Build history of the part. All positions in model axes, mm. A direction names the side the tool comes from. Round coordinates to 2 decimals unless told otherwise and drop trailing zeros. Write each loop counter-clockwise with the first axis right and the second up, starting at its lowest first coordinate (ties: lowest second). Pieces come first, ordered by that corner, then holes. Notation, with made-up numbers: M -1,64 L 40,64 A23 cw 40,82 Z; hole C 15.5,-25.5 d11. An arc over 180 degrees is marked long. Write item = value, one per line. Start each with the question number.
Q1. Band-saw the part on A-A on z = 0. Write the cut outline in (x, y).
Q2. Drop flat-ended pins along their axis: P1, Ø1, axis at x = 7.5, y = -2.5, coming from the -Z side; P2, Ø1.5, axis at x = 16, z = -2, coming from the -Y side; P3, Ø4, axis at x = -12.5, y = -11, coming from the +Z side. Give the stop position or say it passes through.
Q3. Pull direction Y, two halves, no side cores. Call faces 6 (the flat face through (0, 10, 0)), 7 (the cylindrical face through (-15.5, 0.1, 0)), 8 (the cylindrical face through (10.5, 0.1, 0)), 9 (the flat face through (0, 0, -2)): released by +Y, released by -Y, zero draft, split by the parting line, or undercut.
Q4. Tool access for faces 1 (the flat face through (0, 0, 2)), 2 (the flat face through (10, -15, 0)), 3 (the flat face through (-20, -1, 0)), 4 (the flat face through (-10, -15, 0)), 5 (the cylindrical face through (19.715, 9.699, -0.028)): list every direction of +Z, -Z, +X, -X, +Y, -Y with a clear straight run to the whole face (end or side of a thin tool).
Q5. Band-saw the part on C-C on y = 1.5. Write the cut outline in (x, z), plus the area to 3 significant figures.
Q6. Band-saw the part on D-D on x = -8.5. Write the cut outline in (y, z), plus the area to 3 significant figures.
Q7. Band-saw the part on B-B on x = -13. Write the cut outline in (y, z).
Q8. Probe L1, parallel to Y at x = 13, z = 0.15; L2, parallel to Y at x = -3.5, z = 0; L3, parallel to X at y = -1, z = 1.75. List the from-to ranges inside material, lowest first.
```python
from build123d import *

# Parameters (mm, degrees)
SKETCH2_W           = 40
SKETCH2_H           = 20
SKETCH2_R           = 2.5
BOSS_EXTRUDE2_DEPTH = 2
SKETCH5_R           = 3
SKETCH5_R_2         = 2
BOSS_EXTRUDE3_DEPTH = 10
FILLET1_R           = 1


with BuildPart() as part:
    # Sketch2 → Boss-Extrude2 (new body, symmetric)
    with BuildSketch(Plane.XY):
        Rectangle(SKETCH2_W, SKETCH2_H)
        with Locations((-13, 0)):
            Circle(SKETCH2_R, mode=Mode.SUBTRACT)
        with Locations((13, 0)):
            Circle(SKETCH2_R, mode=Mode.SUBTRACT)
    extrude(amount=BOSS_EXTRUDE2_DEPTH, both=True)

    # Sketch5 → Boss-Extrude3 (add, symmetric)
    with BuildSketch(Plane(origin=(0, 0, 0), x_dir=(0, 0, -1), z_dir=(1, 0, 0))):
        with Locations((0, -12.5)):
            Circle(SKETCH5_R)
        with Locations((0, -12.5)):
            Circle(SKETCH5_R_2, mode=Mode.SUBTRACT)
    extrude(amount=BOSS_EXTRUDE3_DEPTH, both=True)

    # Fillet1
    fillet1_edges = [part.edges().sort_by_distance(p)[0] for p in [
        (-20, 10, 0),
        (20, 10, 0),
    ]]
    fillet(fillet1_edges, radius=FILLET1_R)


solid = part.part
```
Conclusion:
q1.outline = M -20,-10 L -10,-10 L -10,-10.5 L 10,-10.5 L 10,-10 L 20,-10 L 20,9 A1 ccw 19,10 L -19,10 A1 ccw -20,9 Z; M -10,-15.5 L 10,-15.5 L 10,-14.5 L -10,-14.5 Z; hole C -13,0 d5; hole C 13,0 d5
q2.P1 = -2
q2.P2 = -10
q2.P3 = 2
q3.face_6 = released by +Y
q3.face_7 = undercut
q3.face_8 = undercut
q3.face_9 = zero draft
q4.face_1 = +Z, +X, -X, +Y
q4.face_2 = +Z, -Z, +X, -Y
q4.face_3 = +Z, -Z, -X, +Y, -Y
q4.face_4 = +Z, -Z, -X, -Y
q4.face_5 = +Z, -Z, +X, +Y
q5.outline = M -20,-2 L -15,-2 L -15,2 L -20,2 Z; M -11,-2 L 11,-2 L 11,2 L -11,2 Z; M 15,-2 L 20,-2 L 20,2 L 15,2 Z
q5.area = 128 mm^2
q6.outline = M -10,-2 L 10,-2 L 10,2 L -10,2 L -10,1.66 A3 ccw long -10,-1.66 Z; hole C -12.5,0 d4
q6.area = 94.6 mm^2
q7.outline = M -10,-2 L -2.5,-2 L -2.5,2 L -10,2 Z; M 2.5,-2 L 10,-2 L 10,2 L 2.5,2 Z
q8.L1 = -10 to -2.5, 2.5 to 10
q8.L2 = -15.5 to -14.5, -10.5 to 10
q8.L3 = -20 to -15.29, -10.71 to 10.71, 15.29 to 20
